Verification items for this drawing (mm, ordinates from the low corner). A direction names the side the tool comes from. Round coordinates to 2 decimals unless told otherwise and drop trailing zeros. Write each loop counter-clockwise with the first axis right and the second up, starting at its lowest first coordinate (ties: lowest second). Pieces come first, ordered by that corner, then holes. Notation, with made-up numbers: (52.5, -15) -> (98.5, -15) arc R18 ccw to (98.5, -9) -> close; hole circle Ø2 at (23, -5.75). An arc over 180 degrees is marked (long way). One line per question, with ' | ' between items.
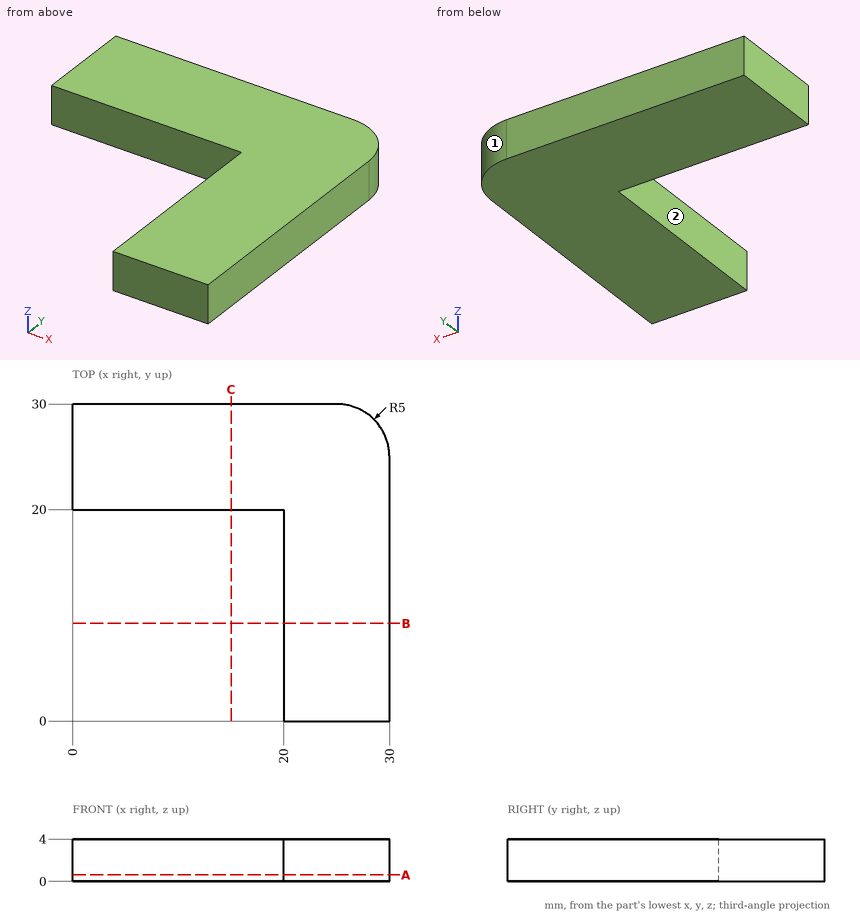
(1) Material ranges on line 1 (Y direction, x = 6.5, z = 1.7); line 2 (Y direction, x = 27.5, z = 0.55), recorded low to high.
Resolved:
line 1: y = 20 to 30 | line 2: y = 0 to 29.33
(2) Sectioned sample at A-A on z = 0.6. Record the cut outline in (x, y).
Resolved:
outline: (0, 20) -> (20, 20) -> (20, 0) -> (30, 0) -> (30, 25) arc R5 ccw to (25, 30) -> (0, 30) -> close
(3) Access from +Z, -Z, +X, -X, +Y, -Y to the whole of each face (thin tool, end or side, straight path). Record for the marked faces 1 and 2.
Resolved:
face 1: +Z, -Z, +X, +Y | face 2: +Z, -Z, -X, -Y
(4) Go/stop test with a flat-tipped pin: pin 1 (1.5 mm diameter, centred on y = 23, z = 2.5, fed in from -X). Record where the tip stops, or that it passes through.
Resolved:
pin 1: stops at x = 0
(5) Sectioned sample at B-B on y = 9.25. Record the cut outline in (x, z).
Resolved:
outline: (20, 0) -> (30, 0) -> (30, 4) -> (20, 4) -> close
